from build123d import *

# Parameters (mm, degrees)
F0_R     = 2.25
F1_DEPTH = 5
F2_SIZE  = 2.5
F3_R     = 4.25
F4_DEPTH = 3


with BuildPart() as f1:
    # F0 (on Top) → F1 (new body)
    with BuildSketch(Plane.XY):
        Polygon((0, 60), (0, 20.5), (20.5, 20.5), (20.5, 0), (60, 0), (60, 20), (20, 60), align=None)
        with Locations((10, 30)):
            Circle(F0_R, mode=Mode.SUBTRACT)
        with Locations((30, 10)):
            Circle(F0_R, mode=Mode.SUBTRACT)
        with Locations((50, 10)):
            Circle(F0_R, mode=Mode.SUBTRACT)
        with Locations((10, 50)):
            Circle(F0_R, mode=Mode.SUBTRACT)
        Polygon((20, 35.142136), (20, 45.857864), (45.857864, 20), (35.142136, 20), align=None, mode=Mode.SUBTRACT)
    extrude(amount=F1_DEPTH)

    # F2
    f2_edges = [f1.edges().sort_by_distance(p)[0] for p in [
        (10.25, 20.5, 5),
        (20.5, 10.25, 5),
        (40.25, 0, 5),
        (60, 10, 5),
        (40, 40, 5),
        (10, 60, 5),
        (0, 40.25, 5),
        (20, 40.5, 5),
        (32.928932, 32.928932, 5),
        (40.5, 20, 5),
        (27.571068, 27.571068, 5),
    ]]
    chamfer(f2_edges, length=F2_SIZE)

    # F3 (on face) → F4 (cut)
    with BuildSketch(Plane.XY.offset(5)):
        with Locations((10, 50)):
            Circle(F3_R)
        with Locations((10, 30)):
            Circle(F3_R)
        with Locations((30, 10)):
            Circle(F3_R)
        with Locations((50, 10)):
            Circle(F3_R)
    extrude(amount=-F4_DEPTH, mode=Mode.SUBTRACT)


solid = f1.part
Source: CAD feature listing. Evaluate the final solid. Frame: model axes, mm. A direction names the side the tool comes from. Coordinates: 2 decimals unless noted, no trailing zeros. Order: outer loops, then holes, each group sorted by start corner. A loop starts at its lowest first (then second) coordinate and runs counter-clockwise, first axis right, second up. Notation, with made-up numbers: M 6.25,-14 L 35.25,-14 A24 cw 35.25,22 Z; hole C 33,82.25 d6. An arc over 180 degrees is marked long. Write each question's results on one line, items separated by ' | '. Start each with the question number.
1. Section A-A, the plane y = 10. Return the cut outline in (x, z), then the cut area to 3 significant figures.
2. Section D-D, the plane y = 41. Return the cut outline in (x, z), then the cut area to 3 significant figures.
3. Draft query along X for faces 4 (the face through (10.1, 58.7, 3.8)), 5 (the face through (1.3, 40.5, 3.8)), 6 (the face through (52, 8, 2)). Return one class per face: +X half, -X half, draft (parallel to the pull), parting line (faces both ways), or undercut.
4. Reachability of faces 1 (the face through (9.08, 45.85, 3.52)), 2 (the face through (10, 20.5, 1)), 3 (the face through (32.75, 33.11, 1.23)) from +Z, -Z, +X, -X, +Y, -Y: full face, straight path, thin tool, end or side. Return the list, or none.
5. Section B-B, the plane z = 0.95. Return the cut outline in (x, y).
6. Material intervals for L1, parallel to Y at x = 10, z = 1.6; L2, parallel to Y at x = 30, z = 0.8, sorted ascending.
7. Pin query (flat end, axial travel): pin 1 (2 mm diameter, centred on x = 9.5, z = 2, fed in from -Y); pin 2 (2.5 mm diameter, centred on x = 12, y = 48.5, fed in from +Z); pin 3 (1.5 mm diameter, centred on y = 12, z = 4, fed in from +X). Return the tip coordinate at first contact, or that it passes through.
Solution:
1) outline: M 20.5,0 L 27.75,0 L 27.75,2 L 25.75,2 L 25.75,5 L 23,5 L 20.5,2.5 Z; M 32.25,0 L 47.75,0 L 47.75,2 L 45.75,2 L 45.75,5 L 34.25,5 L 34.25,2 L 32.25,2 Z; M 52.25,0 L 60,0 L 60,2.5 L 57.5,5 L 54.25,5 L 54.25,2 L 52.25,2 Z | area: 122 mm²
2) outline: M 0,0 L 20,0 L 20,2.5 L 17.5,5 L 2.5,5 L 0,2.5 Z; M 24.86,0 L 39,0 L 39,2.5 L 35.46,5 L 28.39,5 L 24.86,2.5 Z | area: 156 mm²
3) face 4: draft | face 5: -X half | face 6: undercut
4) face 1: +Z | face 2: +Z, -Z, -X, -Y | face 3: +Z, -Z
5) outline: M 0,20.5 L 20.5,20.5 L 20.5,0 L 60,0 L 60,20 L 20,60 L 0,60 Z; hole C 10,30 d4.5; hole C 10,50 d4.5; hole M 20,35.14 L 35.14,20 L 45.86,20 L 20,45.86 Z; hole C 30,10 d4.5; hole C 50,10 d4.5
6) L1: 20.5 to 27.75, 32.25 to 47.75, 52.25 to 60 | L2: 0 to 7.75, 12.25 to 25.14, 35.86 to 50
7) pin 1: y = 20.5 | pin 2: z = 2 | pin 3: x = 59.25
